from build123d import *

# Parameters (mm, degrees)
SKETCH1_W           = 95
SKETCH1_H           = 83.5
SKETCH1_W_2         = 89
SKETCH1_H_2         = 77.5
BOSS_EXTRUDE1_DEPTH = 3
SKETCH1_3_W         = 95
SKETCH1_3_H         = 83.5
SKETCH1_3_W_2       = 89
SKETCH1_3_H_2       = 77.5
BOSS_EXTRUDE2_DEPTH = 17
CUT_EXTRUDE1_REACH  = 97
SKETCH2_W           = 6
SKETCH2_H           = 6
FILLET1_R           = 3


with BuildPart() as part:
    # Sketch1 → Boss-Extrude1 (new body)
    with BuildSketch(Plane(origin=(0, 0, 0), x_dir=(1, 0, 0), z_dir=(0, 1, 0))):
        Rectangle(SKETCH1_W, SKETCH1_H)
        Rectangle(SKETCH1_W_2, SKETCH1_H_2, mode=Mode.SUBTRACT)
        Rectangle(SKETCH1_W_2, SKETCH1_H_2)
    extrude(amount=BOSS_EXTRUDE1_DEPTH)

    # Sketch1_3 → Boss-Extrude2 (add)
    with BuildSketch(Plane(origin=(0, 0, 0), x_dir=(1, 0, 0), z_dir=(0, 1, 0))):
        Rectangle(SKETCH1_3_W, SKETCH1_3_H)
        Rectangle(SKETCH1_3_W_2, SKETCH1_3_H_2, mode=Mode.SUBTRACT)
    extrude(amount=BOSS_EXTRUDE2_DEPTH)

    # Sketch2 → Cut-Extrude1 (cut, up to next)
    with BuildSketch(Plane(origin=(47.5, 0, 0), x_dir=(0, 0, -1), z_dir=(1, 0, 0)), mode=Mode.PRIVATE) as cut_extrude1_sk1:
        with Locations((-32.75, 14)):
            Rectangle(SKETCH2_W, SKETCH2_H)
    cut_extrude1_tool1 = extrude(cut_extrude1_sk1.sketch, amount=-CUT_EXTRUDE1_REACH, mode=Mode.PRIVATE) & part.part
    add(cut_extrude1_tool1.solids().sort_by_distance((47.5, 14, 32.75))[0], mode=Mode.SUBTRACT)
    # Sketch2 → Cut-Extrude1 (cut, up to next)
    with BuildSketch(Plane(origin=(47.5, 0, 0), x_dir=(0, 0, -1), z_dir=(1, 0, 0)), mode=Mode.PRIVATE) as cut_extrude1_sk2:
        with Locations((1.25, 14)):
            Rectangle(SKETCH2_W, SKETCH2_H)
    cut_extrude1_tool2 = extrude(cut_extrude1_sk2.sketch, amount=-CUT_EXTRUDE1_REACH, mode=Mode.PRIVATE) & part.part
    add(cut_extrude1_tool2.solids().sort_by_distance((47.5, 14, -1.25))[0], mode=Mode.SUBTRACT)

    # Fillet1
    fillet1_edges = [part.edges().sort_by_distance(p)[0] for p in [
        (-47.5, 0, 0),
        (0, 0, -41.75),
        (47.5, 0, 0),
        (0, 0, 41.75),
        (-47.5, 8.5, 41.75),
        (-47.5, 8.5, -41.75),
        (47.5, 8.5, -41.75),
        (47.5, 8.5, 41.75),
    ]]
    fillet(fillet1_edges, radius=FILLET1_R)


solid = part.part
Could you check a few things on this model? Use its own coordinates, in mm. A direction names the side the tool comes from. Give positions to 0.01 mm unless a question says otherwise; leave off trailing zeros. Write each loop counter-clockwise with the first axis right and the second up, starting at its lowest first coordinate (ties: lowest second). Pieces come first, ordered by that corner, then holes. Notation, with made-up numbers: (46, 37.5) -> (68, 37.5) arc R16 ccw to (68, 54.5) -> close; hole circle Ø7 at (87.25, 77.25). An arc over 180 degrees is marked (long way). Answer as a JSON object with one key per item and string values.
Q1. Suppose I cut it at C-C on z = 18.5. Write out the boundary of the cut face in (x, y), then the cut area to 3 significant figures.
Taken from the geometry:
{"outline": "(-47.5, 3) arc R3 ccw to (-44.5, 0) -> (44.5, 0) arc R3 ccw to (47.5, 3) -> (47.5, 17) -> (44.5, 17) -> (44.5, 3) -> (-44.5, 3) -> (-44.5, 17) -> (-47.5, 17) -> close", "area": "365 mm²"}
Q2. Will these pins go through, and if not, where does the flat tip stop? pin 1 Ø2.5 at (x, y) = (46, 13) entering from -Z; pin 2 Ø1.5 at (x, z) = (46.5, -1.5) entering from +Y; pin 3 Ø1.5 at (x, y) = (45.5, 15.5) entering from +Z.
Taken from the geometry:
{"pin 1": "stops at z = -41.74", "pin 2": "stops at y = 11", "pin 3": "stops at z = 41.74"}
Q3. Suppose I cut it at A-A on y = 6.25. Write out the boundary of the cut face in (x, z), then the cut area to 3 significant figures.
Taken from the geometry:
{"outline": "(-47.5, -38.75) arc R3 ccw to (-44.5, -41.75) -> (44.5, -41.75) arc R3 ccw to (47.5, -38.75) -> (47.5, 38.75) arc R3 ccw to (44.5, 41.75) -> (-44.5, 41.75) arc R3 ccw to (-47.5, 38.75) -> close; hole (-44.5, -38.75) -> (44.5, -38.75) -> (44.5, 38.75) -> (-44.5, 38.75) -> close", "area": "1,030 mm²"}
Q4. Please list where these lines run through material, in increasing order: L1, parallel to Z at x = 30, y = 12.75; L2, parallel to X at y = 12.5, z = 2; L3, parallel to Y at x = -42, z = 7.
Taken from the geometry:
{"L1": "z = -41.75 to -38.75, 38.75 to 41.75", "L2": "x = -47.5 to -44.5, 44.5 to 47.5", "L3": "y = 0 to 3"}
Q5. We'd pull the mould along X, two halves only. Please class faces 1 (the flat face through (-1, 10, -38.75)), 2 (the cylindrical face through (-46.64, 10.1, 40.85)), 3 (the cylindrical face through (46.6, 9.9, -40.89)): released by +X, released by -X, zero draft, split by the parting line, or undercut.
Taken from the geometry:
{"face 1": "undercut", "face 2": "released by -X", "face 3": "released by +X"}
Q6. Which directions (+Z, -Z, +X, -X, +Y, -Y) give clear straight access to the entire face, cutting with the end or side of a thin tool? Please do faces 4 (the flat face through (46, 14, 29.75)), 5 (the flat face through (44.5, 10, 1)), 6 (the flat face through (-47.5, 10, 1)).
Taken from the geometry:
{"face 4": "+X, +Y", "face 5": "+Y", "face 6": "+Z, -Z, -X, +Y, -Y"}
Q7. Suppose I cut it at B-B on x = 38. Write out the boundary of the cut face in (y, z), then the cut area to 3 significant figures.
Taken from the geometry:
{"outline": "(0, -38.75) arc R3 ccw to (3, -41.75) -> (17, -41.75) -> (17, -38.75) -> (3, -38.75) -> (3, 38.75) -> (17, 38.75) -> (17, 41.75) -> (3, 41.75) arc R3 ccw to (0, 38.75) -> close", "area": "331 mm²"}
